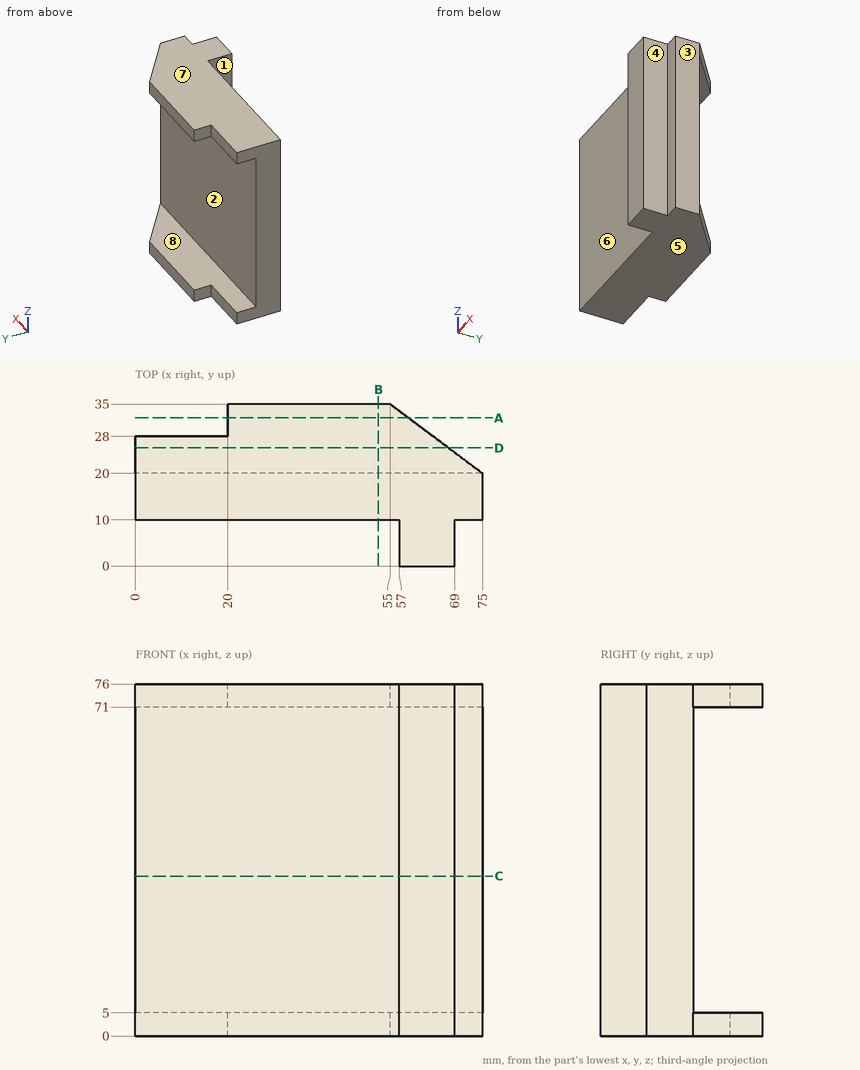
Source: three-view drawing plus pictorial views. Frame: mm from the lowest corner of the part. A direction names the side the tool comes from. Round coordinates to 2 decimals unless told otherwise and drop trailing zeros. Loops run counter-clockwise (first coordinate to the right, second up) from the corner with the lowest first, then second, coordinate; pieces in that order, holes last. Notation, with made-up numbers: M -27,-18.75 L -12,-18.75 A22 cw -12,11.25 Z; hole C -32,-6.5 d10. An arc over 180 degrees is marked long. Answer as CSV lines item,"result". Start each with the question number.
(1) Section A-A, the plane y = 32. Output: boundary loops of the cut face in (x, z).
(2) Section B-B, the plane x = 52.5. Output: boundary loops of the cut face in (y, z), plus the area to 3 significant figures.
(3) Draft query along Z for the marked faces 5, 6, 7 and 8. Return one class per face: released by +Z, released by -Z, zero draft, split by the parting line, or undercut.
(4) Section D-D, the plane y = 25.5. Output: boundary loops of the cut face in (x, z).
(5) Line query: line 1 (Z direction, x = 45, y = 33.5); line 2 (Y direction, x = 11.5, z = 40.5); line 3 (Y direction, x = 63, z = 65.5). Output: solid intervals per line, ascending. Write a range as [from, to].
(6) Section C-C, the plane z = 34.5. Output: boundary loops of the cut face in (x, y), plus the area to 3 significant figures.
(7) Reachability of the marked faces 1, 2, 3 and 4 from +Z, -Z, +X, -X, +Y, -Y: full face, straight path, thin tool, end or side. Return the list, or none.
(8) First-contact query: pin 1 (20 mm diameter, centred on x = 30.5, z = 49, fed in from +Y); pin 2 (2 mm diameter, centred on y = 5.5, z = 52, fed in from -X); pin 3 (1.5 mm diameter, centred on y = 32, z = 73.5, fed in from -X); pin 4 (12 mm diameter, centred on y = 6.5, z = 34, fed in from +X). Flat tips, straight axial feed; report the tip coordinate or a pass-through.
Values found:
1,outline,"M 20,0 L 59,0 L 59,5 L 20,5 Z; M 20,71 L 59,71 L 59,76 L 20,76 Z"
2,outline,"M 10,0 L 35,0 L 35,5 L 20,5 L 20,71 L 35,71 L 35,76 L 10,76 Z"
2,area,"910 mm²"
3,face 5,"released by -Z"
3,face 6,"zero draft"
3,face 7,"released by +Z"
3,face 8,"undercut"
4,outline,"M 0,0 L 67.67,0 L 67.67,5 L 0,5 Z; M 0,71 L 67.67,71 L 67.67,76 L 0,76 Z"
5,line 1,"z = [0, 5], [71, 76]"
5,line 2,"y = [10, 20]"
5,line 3,"y = [0, 20]"
6,outline,"M 0,10 L 57,10 L 57,0 L 69,0 L 69,10 L 75,10 L 75,20 L 0,20 Z"
6,area,"870 mm²"
7,face 1,"+Z, -Z, -X, -Y"
7,face 2,"+X, -X, +Y"
7,face 3,"+Z, -Z, +X, +Y, -Y"
7,face 4,"+Z, -Z, +X, -Y"
8,pin 1,"stops at y = 20"
8,pin 2,"stops at x = 57"
8,pin 3,"stops at x = 20"
8,pin 4,"stops at x = 75"
